For this review, take the finished solid that the model builds, in its own axes (mm). Face numbers are marked on the shaded views. A direction names the side the tool comes from. Coordinates: 2 decimals unless noted, no trailing zeros. Order: outer loops, then holes, each group sorted by start corner. A loop starts at its lowest first (then second) coordinate and runs counter-clockwise, first axis right, second up. Notation, with made-up numbers: M 35,83.5 L 41,83.5 A12 cw 41,101.5 Z; hole C 79.5,51 d9. An arc over 180 degrees is marked long. Use CSV: the item, a comma, the result in double quotes.
Autodesk Inventor part; units mm, degrees
ref_plane "YZ Plane" through (0, 0, 0) normal (1, 0, 0) x (0, 1, 0)
ref_plane "XZ Plane" through (0, 0, 0) normal (0, 1, 0) x (-1, 0, 0)
ref_plane "XY Plane" through (0, 0, 0) normal (0, 0, 1) x (1, 0, 0)
sketch "Sketch1" plane through (0, 0, 0) normal (0, 0, 1) x (1, 0, 0)
  line L0 (-27.7572, -12.1904) -> (-27.7572, 24.8936)
  line L1 (-27.7572, 24.8936) -> (-25.2172, 25.7064)
  line L2 (-25.2172, 25.7064) -> (-19.7562, 21.1241)
  line L3 (8.4378, 24.8936) -> (8.4378, -12.1904)
  line L4 (8.4378, -12.1904) -> (-27.7572, -12.1904)
  line L5 (8.4378, 24.8936) -> (6.093, 25.8702)
  line L6 (0.4368, 21.1241) -> (6.093, 25.8702)
  arc A0 (0.4368, 21.1241) -> (-19.7562, 21.1241) centre (-9.6597, 0.6145) ccw
  point P0 (0, 0)
  dimension "d0" = 37.084
  dimension "d2" = 36.195
  dimension "d3" = 37.084
  dimension "d4" = 50
  dimension "d6" = 37.8968
  dimension "d7" = 2.54
  dimension "d12" = 8.001
  dimension "d13" = 8.001
  dimension "d15" = 2.54
  dimension "d16" = 50
  dimension "d17" = 38.0607
  dimension "d18" = 22.86
extrude "Extrusion1" add sketch "Sketch1" along normal blind 2.54
sketch "Sketch2" plane through (0, 0, 0) normal (0, 0, -1) x (-1, 0, 0)
  line L0 (8.7072, -12.1904) -> (10.6122, -12.1904)
  line L1 (10.6122, -12.1904) -> (10.6122, 17.5276)
  line L2 (10.6122, 17.5276) -> (8.7072, 17.5276)
  line L3 (8.7072, 17.5276) -> (8.7072, -12.1904)
  line L4 (27.7572, 24.8936) -> (27.7572, -12.1904)
  line L5 (27.7572, -12.1904) -> (-8.4378, -12.1904)
  point P0 (0, 0)
  dimension "d21" = 29.718
  dimension "d22" = 1.905
  dimension "d23" = 17.145
  dimension "d24" = 0
extrude "Extrusion2" add sketch "Sketch2" along normal blind 11.43
sketch "Sketch3" plane through (-8.7072, -12.1904, 0) normal (1, 0, 0) x (0, 0, -1)
  line L0 (0, 29.718) -> (11.43, 29.718)
  line L1 (11.43, 29.718) -> (2.54, 29.718)
  line L2 (9.144, 26.543) -> (2.54, 29.718)
  line L3 (11.43, 29.718) -> (11.43, 5.588)
  line L4 (11.43, 5.588) -> (9.144, 26.543)
  point P0 (0, 12.1904)
  dimension "d27" = 8.89
extrude "Extrusion3" cut sketch "Sketch3" against normal through all
sketch "Sketch4" plane through (-27.7572, -12.1904, 2.54) normal (0, -1, 0) x (1, 0, 0)
  line L0 (0, -2.54) -> (0, 0)
  circle A0 centre (4.2418, -1.27) radius 1.27
  line L1 (8.001, 0) -> (2.54, 0)
  point P0 (27.7572, -2.54)
extrude "Extrusion4" add sketch "Sketch4" along normal blind 8.128
sketch "Sketch5" plane through (8.4378, -12.1904, 0) normal (0, -1, 0) x (1, 0, 0)
  circle A0 centre (-4.2418, 1.2916) radius 1.2484
  line L0 (-2.3447, 2.54) -> (-8.001, 2.54)
  point P0 (-8.4378, 0)
extrude "Extrusion5" add sketch "Sketch5" along normal blind 8.128
sketch "Sketch6" plane through (0, 0, 2.54) normal (0, 0, 1) x (1, 0, 0)
  line L0 (-27.7256, 27.1084) -> (8.5248, 27.1084) construction
  line L1 (8.5248, 27.1084) -> (8.5248, -12.2491) construction
  line L2 (8.5248, -12.2491) -> (-27.7256, -12.2491) construction
  line L3 (-27.7256, -12.2491) -> (-27.7256, 27.1084) construction
  point P0 (0, 0)
decal "Decal1"
properties part number "Assignment 4 - Tiger Face [Complete]"
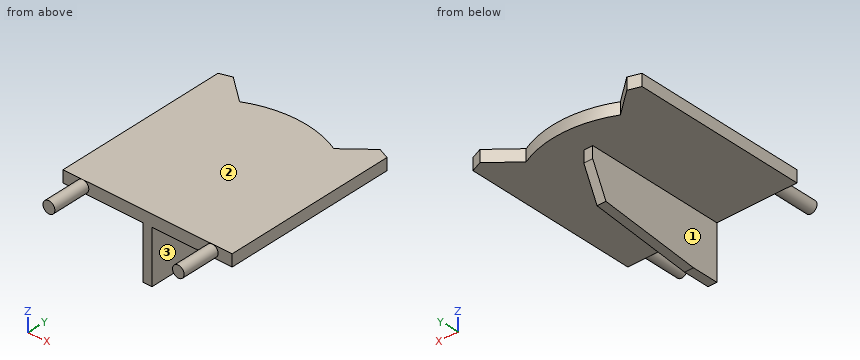
Item 1: Add section C-C on z = -4.5. State the section outline as (x, y) points.
Solutions:
outline,"M -10.61,-12.19 L -8.71,-12.19 L -8.71,16.59 L -10.61,16.59 Z"
Item 2: Add section D-D on y = 13. State the section outline as (x, z) points, and give its area (3 significant figures).
Solutions:
outline,"M -27.76,0 L -10.61,0 L -10.61,-9.29 L -8.71,-9.29 L -8.71,0 L 8.44,0 L 8.44,2.54 L -27.76,2.54 Z"
area,"110 mm^2"
Item 3: For the marked faces 1, 2 and 3, list the 3-axis set-ups (+Z, -Z, +X, -X, +Y, -Y) from which the entire face can be reached by the end or side of a thin tool; tool diameter is ignored.
Solutions:
face 1,"-Z, -X, +Y, -Y"
face 2,"+Z, +X, -X, +Y, -Y"
face 3,"-Z, +X, +Y, -Y"
Item 4: Add section A-A on y = 6. State the section outline as (x, z) points.
Solutions:
outline,"M -27.76,0 L -10.61,0 L -10.61,-10.06 L -8.71,-10.06 L -8.71,0 L 8.44,0 L 8.44,2.54 L -27.76,2.54 Z"
Item 5: Add section B-B on x = 1. State the section outline as (y, z) points, and give its area (3 significant figures).
Solutions:
outline,"M -12.19,0 L 21.6,0 L 21.6,2.54 L -12.19,2.54 Z"
area,"85.8 mm^2"
Item 6: To check wall thickness, follow line 1 along Z through (x, y) = (-1.5, 6); line 2 along X through (y, z) = (-11, -4); line 3 along Z through (x, y) = (-9.5, 8.5). State the ranges of each line that lie inside material, in increasing order. Write a range as [from, to].
Solutions:
line 1,"[0, 2.54]"
line 2,"[-10.61, -8.71]"
line 3,"[-9.78, 2.54]"
Item 7: Clearance check with flat-ended pins moving along their axes: pin 1 Ø1.5 at (x, z) = (-10, -0.5) entering from +Y; pin 2 Ø7 at (x, z) = (-14.5, -2) entering from -Y; pin 3 Ø5 at (x, y) = (-15, -8) entering from -Z. State where each tip first meets the part, or that it passes through.
Solutions:
pin 1,"y = 23.47"
pin 2,"y = -12.19"
pin 3,"z = 0"
